```python
from build123d import *

# Parameters (mm, degrees)
PAD_DEPTH       = 1.7
SKETCH007_W     = 17.37
SKETCH007_H     = 11.44
PAD004_DEPTH    = 4
POCKET002_DEPTH = 5.49
FILLET004_R     = 0.2
FILLET005_R     = 0.2
FILLET006_R     = 0.2
FILLET011_R     = 0.1


with BuildPart() as part:
    # Sketch → Pad (new body)
    with BuildSketch(Plane.XY):
        with BuildLine():
            Line((0, 0), (30, 0))
            Line((30, 0), (30, 1))
            Line((30, 1), (31, 1))
            Line((31, 1), (31, 18.27))
            Line((31, 18.27), (24.4, 18.27))
            ThreePointArc((24.4, 24.87), (21.1, 21.57), (24.4, 18.27))
            Line((24.4, 24.87), (31, 24.87))
            Line((31, 24.87), (31, 59.13))
            Line((31, 59.13), (24.4, 59.13))
            ThreePointArc((24.4, 65.73), (21.1, 62.43), (24.4, 59.13))
            Line((24.4, 65.73), (31, 65.73))
            Line((31, 65.73), (31, 83))
            Line((30, 83), (31, 83))
            Line((30, 84), (30, 83))
            Line((30, 84), (0, 84))
            Line((0, 84), (-30, 84))
            Line((-30, 84), (-30, 83))
            Line((-30, 83), (-31, 83))
            Line((-31, 83), (-31, 65.73))
            Line((-31, 65.73), (-24.4, 65.73))
            ThreePointArc((-24.4, 59.13), (-21.1, 62.43), (-24.4, 65.73))
            Line((-24.4, 59.13), (-31, 59.13))
            Line((-31, 59.13), (-31, 24.87))
            Line((-31, 24.87), (-24.4, 24.87))
            ThreePointArc((-24.4, 18.27), (-21.1, 21.57), (-24.4, 24.87))
            Line((-24.4, 18.27), (-31, 18.27))
            Line((-31, 18.27), (-31, 1))
            Line((-31, 1), (-30, 1))
            Line((-30, 1), (-30, 0))
            Line((-30, 0), (0, 0))
        make_face()
    extrude(amount=PAD_DEPTH)

    # Sketch007 → Pad004 (new body)
    with BuildSketch(Plane.XY.offset(1.7)):
        with Locations((-14.415, 2.72)):
            Rectangle(SKETCH007_W, SKETCH007_H)
    extrude(amount=PAD004_DEPTH)

    # Sketch013 → Pocket002 (cut)
    with BuildSketch(Plane.XZ.offset(3)):
        Polygon((-23.1, 5.7), (-23.1, 4.89), (-21.13, 4.89), (-21.13, 1.7), (-7.85, 1.7), (-7.85, 2.75), (-6.78, 2.75), (-6.78, 4.65), (-7.85, 4.65), (-7.85, 5.7), align=None)
        Polygon((-19.93, 2.7), (-19.93, 4.92), (-9.53, 4.92), (-9.53, 3.67), (-18.74, 3.67), (-18.74, 2.7), align=None, mode=Mode.SUBTRACT)
    extrude(amount=-POCKET002_DEPTH, mode=Mode.SUBTRACT)

    # Fillet004
    fillet004_edges = [part.edges().sort_by_distance(p)[0] for p in [
        (-5.73, 2.72, 5.7),
    ]]
    fillet(fillet004_edges, radius=FILLET004_R)

    # Fillet005
    fillet005_edges = [part.edges().sort_by_distance(p)[0] for p in [
        (-23.1, 5.465, 5.7),
    ]]
    fillet(fillet005_edges, radius=FILLET005_R)

    # Fillet006
    fillet006_edges = [part.edges().sort_by_distance(p)[0] for p in [
        (-23.1, -0.255, 4.89),
    ]]
    fillet(fillet006_edges, radius=FILLET006_R)

    # Fillet011
    fillet011_edges = [part.edges().sort_by_distance(p)[0] for p in [
        (-21.13, -0.255, 4.89),
        (-19.335, -3, 2.7),
        (-19.93, -3, 3.81),
        (-14.73, -3, 4.92),
        (-9.53, -3, 4.295),
        (-14.135, -3, 3.67),
        (-18.74, -3, 3.185),
    ]]
    fillet(fillet011_edges, radius=FILLET011_R)


solid = part.part
```
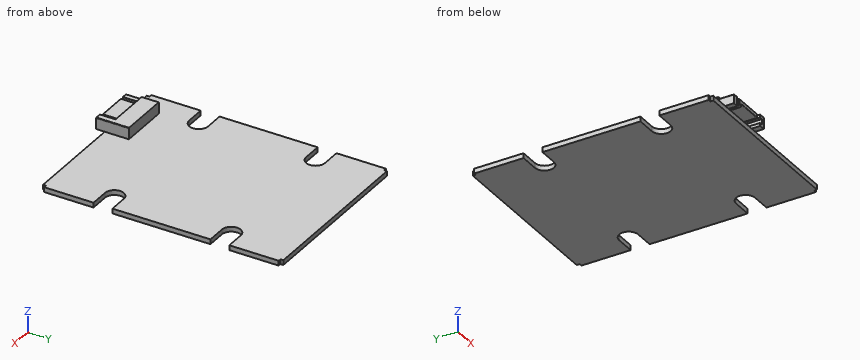
Geometry check sheet. Reference: the model listing, model coordinates, mm. Give positions to 0.01 mm unless a question says otherwise; leave off trailing zeros. Order: outer loops, then holes, each group sorted by start corner. A loop starts at its lowest first (then second) coordinate and runs counter-clockwise, first axis right, second up. Notation, with made-up numbers: (89, 67.5) - (133, 67.5) arc R18 ccw to (133, 74.5) - close; hole circle Ø1 at (65, -9.75). An arc over 180 degrees is marked (long way). Write item = value, one per line. Start each with the question number.
1) Section check D-D (y = 62.43). Enter the section's corners in (x, z), then the cut area to 3 significant figures.
2) Section check A-A (y = 5). Enter the section's corners in (x, z), then the cut area to 3 significant figures.
3) Section check B-B (x = -17.5). Enter the section's corners in (y, z).
4) Gauge pin test, flat ends, axial feed: pin 1 Ø0.5 at (x, z) = (-30.5, 1.5) entering from -Y; pin 2 Ø1.9 at (x, z) = (29, 1) entering from -Y; pin 3 Ø8 at (x, y) = (20.5, 50.5) entering from +Z; pin 4 Ø2 at (y, z) = (26.5, 2.5) entering from +X. Record the tip position at first contact, or that the pin passes through.
5) Section check C-C (x = 19). Enter the section's corners in (y, z), then the cut area to 3 significant figures.
6) Scan lines: L1, parallel to Y at x = -7.5, z = 1.65; L2, parallel to Z at x = 2, y = 70; L3, parallel to Y at x = -23, z = 1.9. Record each from-to range of solid material in increasing order.
Geometry check:
q1.outline = (-21.1, 0) - (21.1, 0) - (21.1, 1.7) - (-21.1, 1.7) - close
q1.area = 71.7 mm2
q2.outline = (-31, 0) - (31, 0) - (31, 1.7) - (-5.73, 1.7) - (-5.73, 5.5) arc R0.2 ccw to (-5.93, 5.7) - (-22.9, 5.7) arc R0.2 ccw to (-23.1, 5.5) - (-23.1, 1.7) - (-31, 1.7) - close
q2.area = 175 mm2
q3.outline = (-3, 3.77) arc R0.1 ccw to (-2.9, 3.67) - (2.49, 3.67) - (2.49, 1.7) - (0, 1.7) - (0, 0) - (84, 0) - (84, 1.7) - (8.44, 1.7) - (8.44, 5.7) - (2.49, 5.7) - (2.49, 4.92) - (-2.9, 4.92) arc R0.1 ccw to (-3, 4.82) - close
q4.pin_1 = 1
q4.pin_2 = 0
q4.pin_3 = 1.7
q4.pin_4 = 31
q5.outline = (0, 0) - (84, 0) - (84, 1.7) - (0, 1.7) - close
q5.area = 143 mm2
q6.L1 = 0 to 84
q6.L2 = 0 to 1.7
q6.L3 = -3 to 8.44
